Geometry check sheet. Reference: the model listing, model coordinates, mm. A direction names the side the tool comes from. Coordinates: 2 decimals unless noted, no trailing zeros. Write each loop counter-clockwise with the first axis right and the second up, starting at its lowest first coordinate (ties: lowest second). Pieces come first, ordered by that corner, then holes. Notation, with made-up numbers: M -20,-8 L -8,-8 A21 cw -8,25 Z; hole C 38.25,53 d5. An arc over 180 degrees is marked long. Put each result on its own line as item: value. Start each with the question number.
1) Cross-section at B-B on y = -33.5. Record the cut outline in (x, z), plus the area to 3 significant figures.
2) Scan lines: line 1 along Y through (x, z) = (43.5, 10); line 2 along X through (y, z) = (-4, 6.5). Record each from-to range of solid material in increasing order.
3) Set-up check for faces 4 (the flat face through (-1, 1, 0)), 5 (the flat face through (1, -56.388, 9)): record each of +Z, -Z, +X, -X, +Y, -Y from which the full face is reachable in a straight line by a thin tool's end or side.
4) Gauge pin test, flat ends, axial feed: pin 1 (4.5 mm diameter, centred on x = -59.944, y = 0, fed in from -Z); pin 2 (2 mm diameter, centred on x = -39, y = -27, fed in from +Z); pin 3 (2 mm diameter, centred on x = 24, y = 33.5, fed in from +Z); pin 4 (1.5 mm diameter, centred on x = -44, y = -23.5, fed in from -Z). Record the tip position at first contact, or that the pin passes through.
5) Cross-section at A-A on z = 10.75. Record the cut outline in (x, y).
6) Cross-section at C-C on x = -19.5. Record the cut outline in (y, z).
7) Cross-section at D-D on x = -2. Record the cut outline in (y, z).
8) Mould release check, pull along Y, two halves, no side actions. Record for faces 1 (the flat face through (-63.5, 1, 6)), 2 (the flat face through (-56.388, -1, 9)), 3 (the flat face through (1, 63.5, 6)): released by +Y, released by -Y, zero draft, split by the parting line, or undercut.
from build123d import *

# Parameters (mm, degrees)
F1_DEPTH = 12.7
F2_DEPTH = 5.08
F3_DEPTH = 7.62
F4_DEPTH = 5.08
F6_DEPTH = 25.4


with BuildPart() as f1:
    # F0 (on Top) → F1 (new body)
    with BuildSketch(Plane.XY):
        Polygon((56.388, -56.388), (0, -56.388), (0, -63.5), (63.5, -63.5), (63.5, 0), (56.388, 0), align=None)
        Polygon((0, -63.5), (0, -56.388), (-56.388, -56.388), (-56.388, 0), (-56.388, 56.388), (0, 56.388), (0, 63.5), (-63.5, 63.5), (-63.5, 0), (-63.5, -63.5), align=None)
        Polygon((0, 63.5), (0, 56.388), (56.388, 56.388), (56.388, 0), (63.5, 0), (63.5, 63.5), align=None)
    extrude(amount=F1_DEPTH)

    # F0 (on Top) → F2 (join)
    with BuildSketch(Plane.XY):
        with BuildLine():
            ThreePointArc((-47.9661298667, 0), (-28.400414984, 22.1775554869), (0, 30.4284702836))
            Line((0, 30.4284702836), (0, 56.388))
            Line((0, 56.388), (-56.388, 56.388))
            Line((-56.388, 56.388), (-56.388, 0))
            Line((-56.388, 0), (-47.9661298667, 0))
        make_face()
        with BuildLine():
            Line((0, 56.388), (0, 30.4284702836))
            ThreePointArc((0, 30.4284702836), (28.4104578527, 22.1822105281), (47.9835120713, 0))
            Line((47.9835120713, 0), (56.388, 0))
            Line((56.388, 0), (56.388, 56.388))
            Line((56.388, 56.388), (0, 56.388))
        make_face()
        with BuildLine():
            Line((52.9104024172, -26.3461358845), (0, -26.3461358845))
            Line((0, -26.3461358845), (0, -56.388))
            Line((0, -56.388), (56.388, -56.388))
            Line((56.388, -56.388), (56.388, 0))
            Line((56.388, 0), (47.9835120713, 0))
            ThreePointArc((47.9835120713, 0), (52.1388015032, -12.8566826028), (52.9104024172, -26.3461358845))
        make_face()
        with BuildLine():
            Line((0, -56.388), (0, -26.3461358845))
            Line((0, -26.3461358845), (-52.8930202127, -26.3461358845))
            ThreePointArc((-52.8930202127, -26.3461358845), (-52.1214192987, -12.8566826028), (-47.9661298667, 0))
            Line((-47.9661298667, 0), (-56.388, 0))
            Line((-56.388, 0), (-56.388, -56.388))
            Line((-56.388, -56.388), (0, -56.388))
        make_face()
    extrude(amount=F2_DEPTH)

    # F0 (on Top) → F3 (join)
    with BuildSketch(Plane.XY):
        with BuildLine():
            ThreePointArc((-32.5514706385, 0), (-19.2050810918, 15.0924405208), (0, 21.181178901))
            Line((0, 21.181178901), (0, 30.4284702836))
            ThreePointArc((0, 30.4284702836), (-28.400414984, 22.1775554869), (-47.9661298667, 0))
            Line((-47.9661298667, 0), (-32.5514706385, 0))
        make_face()
        with BuildLine():
            Line((0, -26.3461358845), (0, -16.5796671063))
            Line((0, -16.5796671063), (-36.3830365241, -16.5796671063))
            ThreePointArc((-36.3830365241, -16.5796671063), (-35.412685982, -8.0713438506), (-32.5514706385, 0))
            Line((-32.5514706385, 0), (-47.9661298667, 0))
            ThreePointArc((-47.9661298667, 0), (-52.1214192987, -12.8566826028), (-52.8930202127, -26.3461358845))
            Line((-52.8930202127, -26.3461358845), (0, -26.3461358845))
        make_face()
        with BuildLine():
            Line((39.1908325255, -16.5796671063), (0, -16.5796671063))
            Line((0, -16.5796671063), (0, -26.3461358845))
            Line((0, -26.3461358845), (52.9104024172, -26.3461358845))
            ThreePointArc((52.9104024172, -26.3461358845), (52.1388015032, -12.8566826028), (47.9835120713, 0))
            Line((47.9835120713, 0), (35.3592666399, 0))
            ThreePointArc((35.3592666399, 0), (38.2204819834, -8.0713438506), (39.1908325255, -16.5796671063))
        make_face()
        with BuildLine():
            Line((0, 30.4284702836), (0, 21.181178901))
            ThreePointArc((0, 21.181178901), (20.8219345928, 15.8362591598), (35.3592666399, 0))
            Line((35.3592666399, 0), (47.9835120713, 0))
            ThreePointArc((47.9835120713, 0), (28.4104578527, 22.1822105281), (0, 30.4284702836))
        make_face()
    extrude(amount=F3_DEPTH)

    # F0 (on Top) → F4 (join)
    with BuildSketch(Plane.XY):
        with BuildLine():
            Line((-32.5514706385, 0), (0, 0))
            Line((0, 0), (0, 21.181178901))
            ThreePointArc((0, 21.181178901), (-19.2050810918, 15.0924405208), (-32.5514706385, 0))
        make_face()
        with BuildLine():
            Line((0, 21.181178901), (0, 0))
            Line((0, 0), (35.3592666399, 0))
            ThreePointArc((35.3592666399, 0), (20.8219345928, 15.8362591598), (0, 21.181178901))
        make_face()
        with BuildLine():
            Line((35.3592666399, 0), (0, 0))
            Line((0, 0), (0, -16.5796671063))
            Line((0, -16.5796671063), (39.1908325255, -16.5796671063))
            ThreePointArc((39.1908325255, -16.5796671063), (38.2204819834, -8.0713438506), (35.3592666399, 0))
        make_face()
        with BuildLine():
            Line((0, -16.5796671063), (0, 0))
            Line((0, 0), (-32.5514706385, 0))
            ThreePointArc((-32.5514706385, 0), (-35.412685982, -8.0713438506), (-36.3830365241, -16.5796671063))
            Line((-36.3830365241, -16.5796671063), (0, -16.5796671063))
        make_face()
    extrude(amount=F4_DEPTH)

    # F5 (on face) → F6 (cut)
    with BuildSketch(Plane.XY.offset(12.7)):
        with BuildLine():
            ThreePointArc((-62.7227567186, 0), (-59.944, -2.7787567186), (-57.1652432814, 0))
            Line((-57.1652432814, 0), (-62.7227567186, 0))
        make_face()
        with BuildLine():
            Line((-62.7227567186, 0), (-57.1652432814, 0))
            ThreePointArc((-57.1652432814, 0), (-59.944, 2.7787567186), (-62.7227567186, 0))
        make_face()
    extrude(amount=-F6_DEPTH, mode=Mode.SUBTRACT)


solid = f1.part
Answer key:
1. outline: M -63.5,0 L 63.5,0 L 63.5,12.7 L 56.39,12.7 L 56.39,5.08 L -56.39,5.08 L -56.39,12.7 L -63.5,12.7 Z
1. area: 754 mm²
2. line 1: y = -63.5 to -56.39, 56.39 to 63.5
2. line 2: x = -63.5 to -56.39, -49.65 to -34.23, 37.04 to 49.67, 56.39 to 63.5
3. face 4: -Z, +X, -X, +Y, -Y
3. face 5: +Z
4. pin 1: passes through
4. pin 2: stops at z = 7.62
4. pin 3: stops at z = 5.08
4. pin 4: stops at z = 0
5. outline: M -63.5,-63.5 L 63.5,-63.5 L 63.5,63.5 L -63.5,63.5 Z; hole C -59.94,0 d5.56; hole M -56.39,-56.39 L 56.39,-56.39 L 56.39,56.39 L -56.39,56.39 Z
6. outline: M -63.5,0 L 63.5,0 L 63.5,12.7 L 56.39,12.7 L 56.39,5.08 L 26.71,5.08 L 26.71,7.62 L 14.9,7.62 L 14.9,5.08 L -16.58,5.08 L -16.58,7.62 L -26.35,7.62 L -26.35,5.08 L -56.39,5.08 L -56.39,12.7 L -63.5,12.7 Z
7. outline: M -63.5,0 L 63.5,0 L 63.5,12.7 L 56.39,12.7 L 56.39,5.08 L 30.39,5.08 L 30.39,7.62 L 21.05,7.62 L 21.05,5.08 L -16.58,5.08 L -16.58,7.62 L -26.35,7.62 L -26.35,5.08 L -56.39,5.08 L -56.39,12.7 L -63.5,12.7 Z
8. face 1: zero draft
8. face 2: undercut
8. face 3: released by +Y
